Here's how the part is built. I have some questions about the finished solid (model axes, mm). A direction names the side the tool comes from. Coordinates: 2 decimals unless noted, no trailing zeros. Write each loop counter-clockwise with the first axis right and the second up, starting at its lowest first coordinate (ties: lowest second). Pieces come first, ordered by that corner, then holes. Notation, with made-up numbers: M 55.25,48.5 L 70.25,48.5 A26 ccw 70.25,64.5 Z; hole C 31.25,31 d6. An arc over 180 degrees is marked long. Use a Markdown table: item, result.
```python
from build123d import *

# Parameters (mm, degrees)
F1_DEPTH = 12.7
F2_T     = -2.54
F3_R     = 3.048


with BuildPart() as f1:
    # F0 (on Top) → F1 (new body, symmetric)
    with BuildSketch(Plane.XY):
        Polygon((25.92500022, -34.52499953), (25.92500022, 34.52499953), (-25.92500022, 34.52499953), (-25.92500022, 28.157905028), (-18.1308021206, 28.157905028), (-18.1308021206, 16.960619828), (-25.92500022, 16.960619828), (-25.92500022, 6.202424428), (-18.1308021206, 6.202424428), (-18.1308021206, -4.9948727434), (-25.92500022, -4.9948727434), (-25.92500022, -15.7530735209), (-18.1308021206, -15.7530735209), (-18.1308021206, -26.9503587209), (-25.92500022, -26.9503587209), (-25.92500022, -34.52499953), align=None)
    extrude(amount=F1_DEPTH, both=True)

    # F2
    f2_openings = [f1.faces().sort_by_distance(p)[0] for p in [
        (1.73799, -0.047637, -12.7),
    ]]
    offset(amount=F2_T, openings=f2_openings, kind=Kind.INTERSECTION)

    # F3
    f3_edges = [f1.edges().sort_by_distance(p)[0] for p in [
        (25.925, 0, 12.7),
        (0, 34.525, 12.7),
        (-25.925, 31.341452, 12.7),
        (-18.130802, 22.559262, 12.7),
        (-22.027901, 16.96062, 12.7),
        (-25.925, 11.581522, 12.7),
        (-22.027901, 6.202424, 12.7),
        (-18.130802, 0.603776, 12.7),
        (-22.027901, -4.994873, 12.7),
        (-25.925, -10.373973, 12.7),
        (-22.027901, -15.753074, 12.7),
        (-18.130802, -21.351716, 12.7),
        (-22.027901, -26.950359, 12.7),
        (-25.925, -30.737679, 12.7),
        (0, -34.525, 12.7),
        (-22.027901, 28.157905, 12.7),
        (-25.925, -34.525, 0),
        (25.925, -34.525, 0),
        (25.925, 34.525, 0),
        (-25.925, 34.525, 0),
    ]]
    fillet(f3_edges, radius=F3_R)


solid = f1.part
```
1. Which directions (+Z, -Z, +X, -X, +Y, -Y) give clear straight access to the entire face, cutting with the end or side of a thin tool? Please do faces 4 (the face through (25.925, 0, -1)), 5 (the face through (-19, 14.421, -1)), 6 (the face through (-18.131, 23, -1)), 7 (the face through (-20.43, 7.07, 11.78)).
Answers follow:
| item | result |
|---|---|
| face 4 | +Z, -Z, +X, +Y, -Y |
| face 5 | -Z |
| face 6 | +Z, -Z, -X |
| face 7 | +Z, -X |
2. We'd pull the mould along Y, two halves only. Please class faces 1 (the face through (0, -34.525, -1)), 2 (the face through (-25.393, -10.449, 11.373)), 3 (the face through (23.385, 0, -1)): +Y half, -Y half, draft (parallel to the pull), parting line (faces both ways), or undercut.
Answers follow:
| item | result |
|---|---|
| face 1 | -Y half |
| face 2 | draft |
| face 3 | undercut |
3. Suppose I cut it at C-C on x = -19. State how many separate pieces and enclosed holes the cut face has, and give its area (3 significant figures).
Answers follow:
| item | result |
|---|---|
| separate pieces | 4 |
| enclosed holes | 0 |
| area | 539 mm2 |
4. Suppose I cut it at D-D on y = 29. Write out the boundary of the cut face in (x, z) (3 decimals), and give its area (3 significant figures).
Answers follow:
| item | result |
|---|---|
| outline | M -25.925,-12.7 L -15.591,-12.7 L -15.591,10.16 L 23.385,10.16 L 23.385,-12.7 L 25.925,-12.7 L 25.925,9.652 A3.048 ccw 22.877,12.7 L -15.083,12.7 A3.048 ccw -17.289,11.755 L -25.083,11.755 A3.048 ccw -25.925,9.652 Z |
| area | 415 mm2 |
5. Suppose I cut it at B-B on x = 2.5. Write out the boundary of the cut face in (y, z) (3 decimals).
Answers follow:
| item | result |
|---|---|
| outline | M -34.525,-12.7 L -31.985,-12.7 L -31.985,10.16 L 31.985,10.16 L 31.985,-12.7 L 34.525,-12.7 L 34.525,9.652 A3.048 ccw 31.477,12.7 L -31.477,12.7 A3.048 ccw -34.525,9.652 Z |
6. Will these pins go through, and if not, where does the flat tip stop? pin 1 Ø5 at (x, y) = (-8.5, -16) entering from -Z; pin 2 Ø3.5 at (y, z) = (0.5, 2.5) entering from -X.
Answers follow:
| item | result |
|---|---|
| pin 1 | stops at z = 10.16 |
| pin 2 | stops at x = -18.13 |
7. Suppose I cut it at A-A on y = -17.5. Write out the boundary of the cut face in (x, z) (3 decimals).
Answers follow:
| item | result |
|---|---|
| outline | M -18.131,-12.7 L -15.591,-12.7 L -15.591,10.16 L 23.385,10.16 L 23.385,-12.7 L 25.925,-12.7 L 25.925,9.652 A3.048 ccw 22.877,12.7 L -15.083,12.7 A3.048 ccw -18.131,9.652 Z |
8. I need wall thicknesses on probe 1 along Y at (x, z) = (-16.5, -3.5) (3 decimals); probe 2 along X at (y, z) = (23, 0.25) (3 decimals); probe 3 along Y at (x, z) = (-10, -10) (3 decimals). Which ranges of each line are inside material? Lowest first, please.
Answers follow:
| item | result |
|---|---|
| probe 1 | y = -34.525 to -31.985, -29.49 to -13.213, -7.535 to 8.742, 14.421 to 30.698, 31.985 to 34.525 |
| probe 2 | x = -18.131 to -15.591, 23.385 to 25.925 |
| probe 3 | y = -34.525 to -31.985, 31.985 to 34.525 |
